Autodesk Inventor part; units mm, degrees
ref_plane "YZ Plane" through (0, 0, 0) normal (1, 0, 0) x (0, 1, 0)
ref_plane "XZ Plane" through (0, 0, 0) normal (0, 1, 0) x (-1, 0, 0)
ref_plane "XY Plane" through (0, 0, 0) normal (0, 0, 1) x (1, 0, 0)
sketch "Sketch6" plane through (0, 0, 0) normal (0, 0, 1) x (1, 0, 0)
  line L0 (0, 0) -> (60, 0)
  line L1 (60, 0) -> (60, 120)
  line L2 (60, 120) -> (0, 120)
  line L3 (0, 120) -> (0, 0)
  dimension "d47" = 60
  dimension "d48" = 120
extrude "Plate3" add sketch "Sketch6" along normal blind 6
sketch "Sketch7" plane through (6, 0, 0) normal (-1, 0, 0) x (0, -1, 0)
  line L0 (-120, 0) -> (0, 0)
  line L1 (0, 0) -> (0, 60)
  line L2 (0, 60) -> (-120, 60)
  line L3 (-120, 60) -> (-120, 0)
edge flange "Flange2" height 60 angle 90 thickness 6 bend radius 5 thickness toward (-1, 0, 0) relief round relief width 6 relief depth 3 edges at (0, 60, 6) wall of the first edge with corners at (6, 120, 0) (6, 0, 0) (6, 0, 60) (6, 120, 60)
bend "Bend2"
corner "Corner2"
equation "\"d46\" = Thickness"
equation "\"d49\" = BendReliefWidth"
equation "\"d50\" = BendReliefDepth"
equation "\"d51\" = MinimumRemnant"
equation "\"d52\" = TransitionRadius"
equation "\"d55\" = BendRadius"
equation "\"d56\" = CornerReliefSize"
equation "\"d57\" = GapSize"
equation "\"d58\" = JacobiRadiusSize"
equation "\"BendReliefWidth\" = Thickness"
equation "\"BendReliefDepth\" = 0.5 * Thickness"
equation "\"CornerReliefSize\" = 4 * Thickness"
equation "\"MinimumRemnant\" = 2 * Thickness"
equation "\"TransitionRadius\" = BendRadius"
equation "\"JacobiRadiusSize\" = BendRadius"
equation "\"GapSize\" = Thickness"
properties part number "GnG frame 4.2 reinf" material "Stainless Steel"
Geometry: final body of the model. Coordinates: model frame, mm. A direction names the side the tool comes from. Give positions to 0.01 mm unless a question says otherwise; leave off trailing zeros. Order: outer loops, then holes, each group sorted by start corner. A loop starts at its lowest first (then second) coordinate and runs counter-clockwise, first axis right, second up. Notation, with made-up numbers: (20.5, 44.25) -> (60.5, 44.25) arc R17 cw to (60.5, 62.25) -> close; hole circle Ø8 at (17.5, -37). An arc over 180 degrees is marked (long way). Answer as a JSON object with one key per item and string values.
Q1. Material intervals for probe 1 along Z at (x, y) = (33, 63); probe 2 along Z at (x, y) = (5, 47.5), sorted ascending.
Entries:
{"probe 1": "z = 0 to 6", "probe 2": "z = 1.78 to 60"}
Q2. Section B-B (z = 12.5). Output: boundary loops of the cut face in (x, y).
Entries:
{"outline": "(0, 0) -> (6, 0) -> (6, 120) -> (0, 120) -> close"}
Q3. First-contact query: pin 1 (1.5 mm diameter, centred on x = 42, y = 79.5, fed in from +Z); pin 2 (2 mm diameter, centred on y = 40.5, z = 35, fed in from +X). Flat tips, straight axial feed; report the tip coordinate or a pass-through.
Entries:
{"pin 1": "stops at z = 6", "pin 2": "stops at x = 6"}
Q4. Section A-A (y = 72.5). Output: boundary loops of the cut face in (x, z).
Entries:
{"outline": "(0, 11) arc R11 ccw to (11, 0) -> (60, 0) -> (60, 6) -> (11, 6) arc R5 cw to (6, 11) -> (6, 60) -> (0, 60) -> close"}
Q5. Access query for faces 1 (the flat face through (6, 59, 35)), 2 (the flat face through (60, 59, 3)). Directions: +Z, -Z, +X, -X, +Y, -Y. A direction counts if a zero-diameter tool reaches every point of the face in a straight line with its end or side. Return the directions, or none.
Entries:
{"face 1": "+Z, +X, +Y, -Y", "face 2": "+Z, -Z, +X, +Y, -Y"}
Q6. Section C-C (x = 54). Output: boundary loops of the cut face in (y, z), plus the area to 3 significant figures.
Entries:
{"outline": "(0, 0) -> (120, 0) -> (120, 6) -> (0, 6) -> close", "area": "720 mm^2"}
